Design review of the part built by this model. Coordinates are the model's own, in mm. Face numbers are marked on the shaded views. Coordinates: 2 decimals unless noted, no trailing zeros. Loops run counter-clockwise (first coordinate to the right, second up) from the corner with the lowest first, then second, coordinate; pieces in that order, holes last.
Q1. Add section D-D on y = -4.5. Give the boundary of the cut face in (x, z).
Q2. Add section B-B on x = 0. Give the boundary of the cut face in (y, z), and give its area (3 significant figures).
Q3. For P1, Ø5, axis at x = -2, z = 12.5, coming from the +Y side; P2, Ø5, axis at x = -3.5, z = 16, coming from the -Y side; P3, Ø5, axis at x = 4, z = 4, coming from the -Y side; P4, Ø1, axis at x = 4, y = 0, coming from the -Z side, all flat-tipped, find the tip position at first contact; note any pin that passes through.
Q4. Wall thickness on probe 1 along X at (y, z) = (0, 8.5); probe 2 along X at (y, z) = (-1.75, 10.5); probe 3 along Y at (x, z) = (0, 16.5): over which ranges is each line inside the solid? List them lowest first.
Q5. Add section A-A on y = -0.75. Give the boundary of the cut face in (x, z), and give its area (3 significant figures).
Q6. Draft analysis for pull direction Y (two halves, no side actions). For the marked faces 1, 2 and 3, state which applies: released by +Y, released by -Y, zero draft, split by the parting line, or undercut.
Q7. Add section C-C on z = 6.5. Give the boundary of the cut face in (x, y).
```python
from build123d import *

# Parameters (mm, degrees)
F1_DEPTH    = 21
F2_T1_DEPTH = 23.8690975764
F2_T3_DEPTH = 30.409576176


# Not quite as in the source:
# - a fillet or chamfer that OpenCascade refuses, or shapes differently, is made with other operations: its cross-section is extruded or revolved along the edge and cut away or added


with BuildPart() as f1:
    # F0 (on Top) → F1 (new body)
    with BuildSketch(Plane.XY):
        with BuildLine():
            ThreePointArc((3.7440062904, 1.6710526316), (4.0100140767, 0.8542757779), (4.1, 0))
            ThreePointArc((4.1, 0), (-0.8542757779, -4.0100140767), (-3.7440062904, 1.6710526316))
            ThreePointArc((-3.7440062904, 1.6710526316), (-4.335673559, 2.3159292575), (-4.8175607103, 3.0464912281))
            ThreePointArc((-4.8175607103, 3.0464912281), (-1.5858600114, -5.4749473079), (5.7, 0))
            ThreePointArc((5.7, 0), (5.4749473079, 1.5858600114), (4.8175607103, 3.0464912281))
            ThreePointArc((4.8175607103, 3.0464912281), (4.335673559, 2.3159292575), (3.7440062904, 1.6710526316))
        make_face()
    extrude(amount=F1_DEPTH)

    # F2: fillet of radius 1 on 4 edges, made by hand

    # F2_s2 → F2_t1 (cut)
    with BuildSketch(Plane.XY.offset(-1.4345487882)):
        with BuildLine():
            ThreePointArc((-4.1434007569, 2.0830634278), (-3.9202406694, 1.6409302608), (-3.9366000062, 1.1459408325))
            ThreePointArc((-3.9366000062, 1.1459408325), (-3.8492679656, 1.4117847318), (-3.7440062904, 1.6710526316))
            ThreePointArc((-3.7440062904, 1.6710526316), (-3.9490803621, 1.8718458373), (-4.1434007569, 2.0830634278))
        make_face()
        with BuildLine():
            ThreePointArc((4.1434007569, 2.0830634278), (3.9202406694, 1.6409302608), (3.9366000062, 1.1459408325))
            ThreePointArc((3.9366000062, 1.1459408325), (3.8492679656, 1.4117847318), (3.7440062904, 1.6710526316))
            ThreePointArc((3.7440062904, 1.6710526316), (3.9490803621, 1.8718458373), (4.1434007569, 2.0830634278))
        make_face()
    extrude(amount=F2_T1_DEPTH, mode=Mode.SUBTRACT)

    # F2_s4 → F2_t3 (cut)
    with BuildSketch(Plane.XY.offset(-4.704788088)):
        with BuildLine():
            ThreePointArc((-5.5470205992, 1.3117021277), (-4.849273554, 2.0429045287), (-3.8701884613, 1.7921052632))
            ThreePointArc((-3.8701884613, 1.7921052632), (-4.3889198505, 2.3852779082), (-4.8175607103, 3.0464912281))
            ThreePointArc((-4.8175607103, 3.0464912281), (-5.2543800525, 2.2094094831), (-5.5470205992, 1.3117021277))
        make_face()
        with BuildLine():
            ThreePointArc((3.8701884613, 1.7921052632), (4.849273554, 2.0429045287), (5.5470205992, 1.3117021277))
            ThreePointArc((5.5470205992, 1.3117021277), (5.2543800525, 2.2094094831), (4.8175607103, 3.0464912281))
            ThreePointArc((4.8175607103, 3.0464912281), (4.3889198505, 2.3852779082), (3.8701884613, 1.7921052632))
        make_face()
    extrude(amount=F2_T3_DEPTH, mode=Mode.SUBTRACT)


solid = f1.part
```
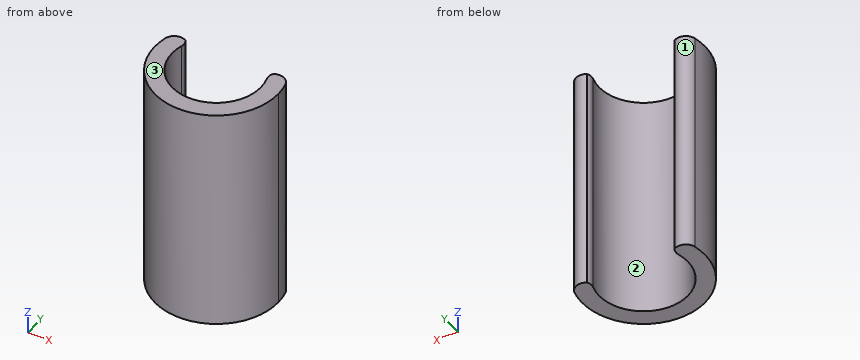
Entries:
1. outline: (-3.5, 0) - (3.5, 0) - (3.5, 21) - (-3.5, 21) - close
2. outline: (-5.7, 0) - (-4.1, 0) - (-4.1, 21) - (-5.7, 21) - close
2. area: 33.6 mm2
3. P1: stops at y = 2.08
3. P2: stops at y = -5.61
3. P3: stops at y = -5.5
3. P4: stops at z = 0
4. probe 1: x = -5.7 to -4.1, 4.1 to 5.7
4. probe 2: x = -5.42 to -3.71, 3.71 to 5.42
4. probe 3: y = -5.7 to -4.1
5. outline: (-5.65, 0) - (-4.03, 0) - (-4.03, 21) - (-5.65, 21) - close; (4.03, 0) - (5.65, 0) - (5.65, 21) - (4.03, 21) - close
5. area: 68.0 mm2
6. face 1: released by +Y
6. face 2: undercut
6. face 3: zero draft
7. outline: (-5.55, 1.31) arc R5.7 ccw (long way) to (5.55, 1.31) arc R1 ccw to (4.03, 1.92) arc R1 ccw to (3.94, 1.15) arc R4.1 cw (long way) to (-3.94, 1.15) arc R1 ccw to (-4.03, 1.92) arc R1 ccw to start
